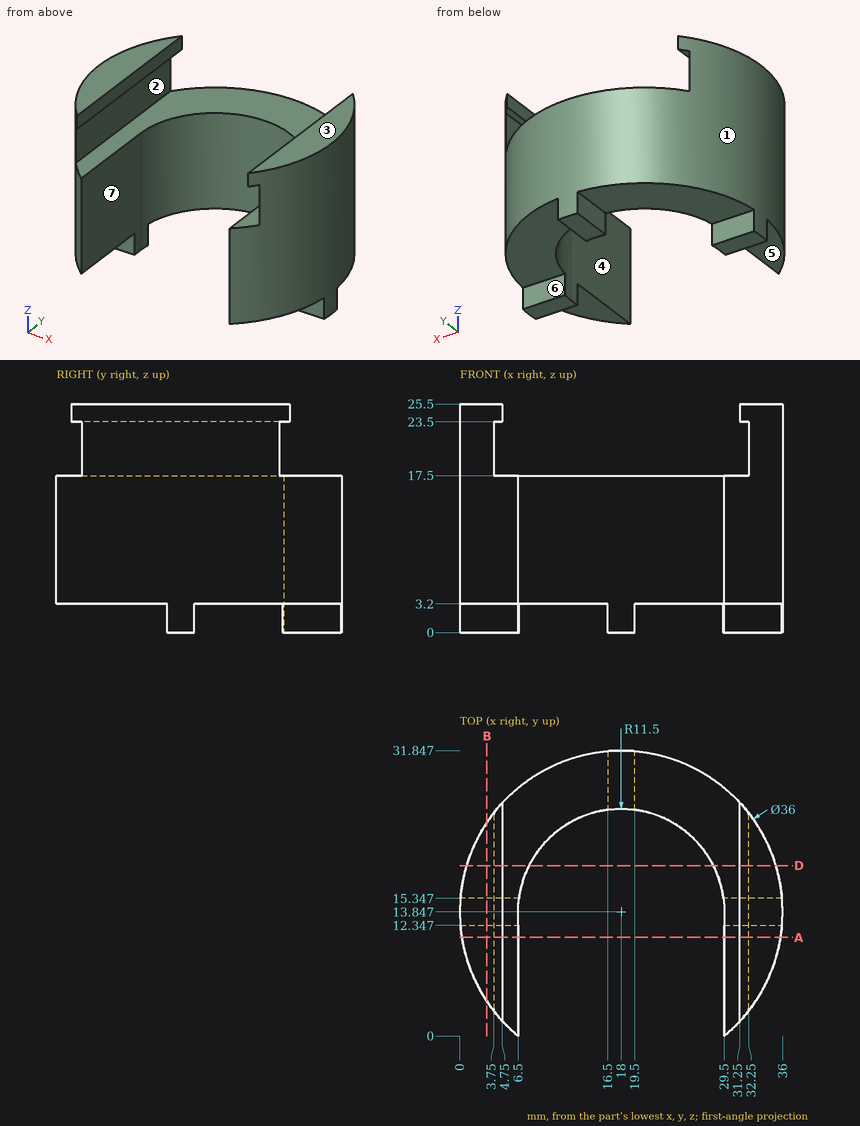
The figure shows three views and two pictorial views of one solid part (mm, origin at its lowest corner). Answer the questions. A direction names the side the tool comes from. Round coordinates to 2 decimals unless told otherwise and drop trailing zeros. Write each loop counter-clockwise with the first axis right and the second up, starting at its lowest first coordinate (ties: lowest second). Pieces come first, ordered by that corner, then holes. Notation, with made-up numbers: M 17,70.25 L 55,70.25 A26 ccw 55,93.25 Z; hole C -4.75,-10 d7. An arc over 180 degrees is marked long. Use a Markdown table: item, result.
1) Flat-ended cylindrical pins translate along their axes: pin 1 (1.6 mm diameter, centred on y = 10, z = 24.5, fed in from -X); pin 2 (1.6 mm diameter, centred on y = 28.5, z = 1.5, fed in from +X); pin 3 (3 mm diameter, centred on x = 3.5, y = 3.5, fed in from -Z); pin 4 (8.5 mm diameter, centred on x = 14.5, y = 14, fed in from +Z). Find the tip coordinate at first contact, or state that the pin passes through.
Taken from the geometry:
| item | result |
|---|---|
| pin 1 | stops at x = 0.26 |
| pin 2 | stops at x = 19.5 |
| pin 3 | stops at z = 3.2 |
| pin 4 | passes through |
2) Consider line 1 (X direction, y = 23, z = 22); line 2 (X direction, y = 7, z = 14); line 3 (Z direction, x = 19, y = 25.5). Determine where each line is inside the solid, lowest interval first. Write a range as [from, to].
Taken from the geometry:
| item | result |
|---|---|
| line 1 | x = [2.5, 3.75], [32.25, 33.5] |
| line 2 | x = [1.35, 6.5], [29.5, 34.65] |
| line 3 | z = [0, 17.5] |
3) The part is cut by section A-A on y = 11. Give the vertices of the cut face in (x, z).
Taken from the geometry:
| item | result |
|---|---|
| outline | M 0.23,3.2 L 6.5,3.2 L 6.5,17.5 L 3.75,17.5 L 3.75,23.5 L 4.75,23.5 L 4.75,25.5 L 0.23,25.5 Z; M 29.5,3.2 L 35.77,3.2 L 35.77,25.5 L 31.25,25.5 L 31.25,23.5 L 32.25,23.5 L 32.25,17.5 L 29.5,17.5 Z |
4) Determine the mould class of the marked faces 1, 2, 3 and 4 for opening direction X: pulls with the +X half, pulls with the -X half, needs draft (parallel to the pull), parting line crosses it, or undercut.
Taken from the geometry:
| item | result |
|---|---|
| face 1 | parting line crosses it |
| face 2 | undercut |
| face 3 | needs draft |
| face 4 | undercut |
5) The part is cut by section D-D on y = 19. Give the vertices of the cut face in (x, z), plus the area to 3 significant figures.
Taken from the geometry:
| item | result |
|---|---|
| outline | M 0.75,3.2 L 7.72,3.2 L 7.72,17.5 L 3.75,17.5 L 3.75,23.5 L 4.75,23.5 L 4.75,25.5 L 0.75,25.5 Z; M 28.28,3.2 L 35.25,3.2 L 35.25,25.5 L 31.25,25.5 L 31.25,23.5 L 32.25,23.5 L 32.25,17.5 L 28.28,17.5 Z |
| area | 251 mm2 |
6) The part is cut by section B-B on x = 3. Give the vertices of the cut face in (y, z).
Taken from the geometry:
| item | result |
|---|---|
| outline | M 3.9,3.2 L 12.35,3.2 L 12.35,0 L 15.35,0 L 15.35,3.2 L 23.8,3.2 L 23.8,25.5 L 3.9,25.5 Z |
7) Which of the six approach directions +Z, -Z, +X, -X, +Y, -Y give full straight-line access (tool end or side, diameter ignored) to the marked faces 5, 6 and 7?
Taken from the geometry:
| item | result |
|---|---|
| face 5 | -Z, +X, -X, -Y |
| face 6 | -Z, +X, -X, +Y |
| face 7 | +Z, -Z, -Y |
